Could you check a few things on this drawing? It's one solid part, dimensions in mm from its lowest x, y, z. Give positions to 0.01 mm unless a question says otherwise; leave off trailing zeros. Loops run counter-clockwise (first coordinate to the right, second up) from the corner with the lowest first, then second, coordinate; pieces in that order, holes last. Notation, with made-up numbers: (83.25, 82) - (125.25, 82) arc R12 cw to (125.25, 97) - close; hole circle Ø5 at (-25.75, 81). An arc over 180 degrees is marked (long way). Use a Markdown table: item, result.
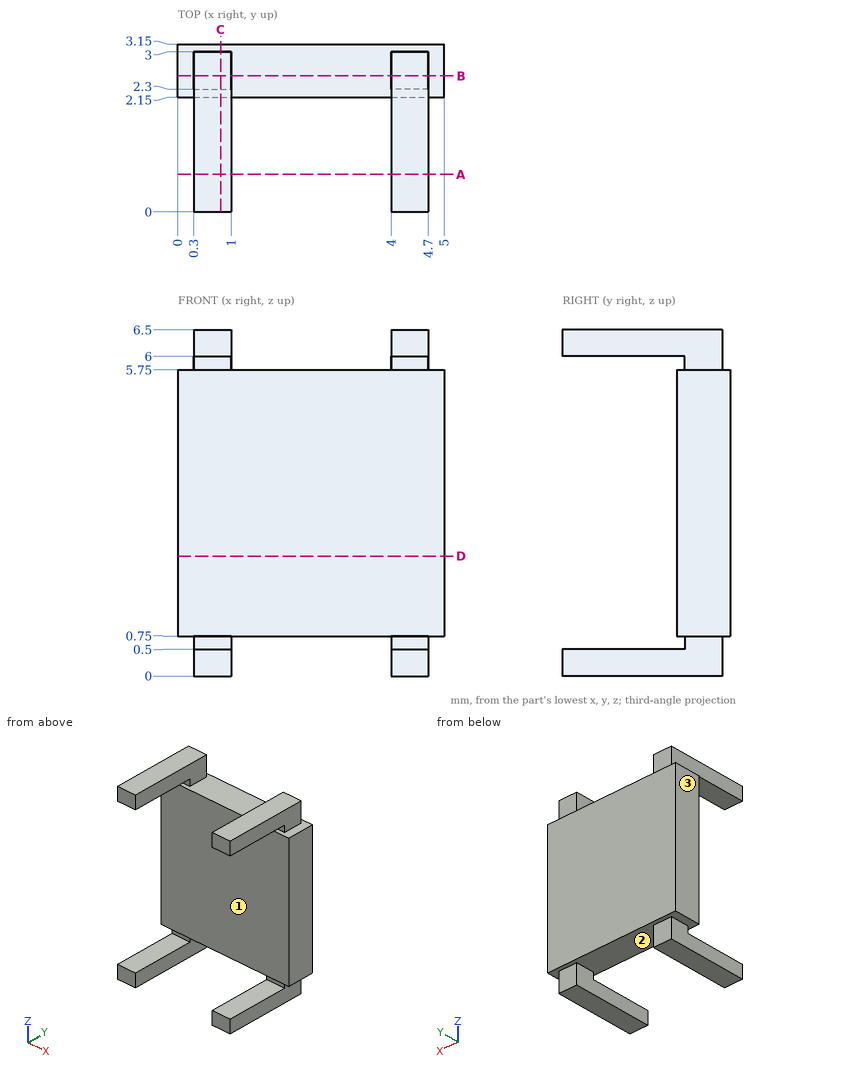
(1) If I drill on line 1 (X direction, y = 2.5, z = 6); line 2 (Y direction, x = 1.2, z = 3); line 3 (Z direction, x = 3.9, y = 2.2), over which ranges is the centre line in solid material (lowest first)?
A:
| item | result |
|---|---|
| line 1 | 0.3 to 1, 4 to 4.7 |
| line 2 | 2.15 to 3.15 |
| line 3 | 0.75 to 5.75 |
(2) We'd pull the mould along X, two halves only. Please class the marked faces 1, 2 and 3: pulls with the +X half, pulls with the -X half, needs draft (parallel to the pull), parting line crosses it, or undercut.
A:
| item | result |
|---|---|
| face 1 | needs draft |
| face 2 | undercut |
| face 3 | pulls with the -X half |
(3) Suppose I cut it at A-A on y = 0.7. Write out the boundary of the cut face in (x, z), plus the area to 3 significant figures.
A:
| item | result |
|---|---|
| outline | (0.3, 0) - (1, 0) - (1, 0.5) - (0.3, 0.5) - close; (0.3, 6) - (1, 6) - (1, 6.5) - (0.3, 6.5) - close; (4, 0) - (4.7, 0) - (4.7, 0.5) - (4, 0.5) - close; (4, 6) - (4.7, 6) - (4.7, 6.5) - (4, 6.5) - close |
| area | 1.40 mm2 |
(4) Suppose I cut it at D-D on z = 2.25. Write out the boundary of the cut face in (x, y), plus the area to 3 significant figures.
A:
| item | result |
|---|---|
| outline | (0, 2.15) - (5, 2.15) - (5, 3.15) - (0, 3.15) - close |
| area | 5.00 mm2 |
(5) Suppose I cut it at C-C on x = 0.8. Write out the boundary of the cut face in (y, z).
A:
| item | result |
|---|---|
| outline | (0, 0) - (3, 0) - (3, 0.75) - (3.15, 0.75) - (3.15, 5.75) - (3, 5.75) - (3, 6.5) - (0, 6.5) - (0, 6) - (2.3, 6) - (2.3, 5.75) - (2.15, 5.75) - (2.15, 0.75) - (2.3, 0.75) - (2.3, 0.5) - (0, 0.5) - close |
(6) Will this pin go through, and if not, where does the flat tip stop? pin 1 (1.5 mm diameter, centred on x = 2.5, z = 1.5, fed in from -Y).
A:
| item | result |
|---|---|
| pin 1 | y = 2.15 |
(7) Suppose I cut it at B-B on y = 2.55. Write out the boundary of the cut face in (x, z).
A:
| item | result |
|---|---|
| outline | (0, 0.75) - (0.3, 0.75) - (0.3, 0) - (1, 0) - (1, 0.75) - (4, 0.75) - (4, 0) - (4.7, 0) - (4.7, 0.75) - (5, 0.75) - (5, 5.75) - (4.7, 5.75) - (4.7, 6.5) - (4, 6.5) - (4, 5.75) - (1, 5.75) - (1, 6.5) - (0.3, 6.5) - (0.3, 5.75) - (0, 5.75) - close |
